Geometry: final body of the model. Coordinates: model frame, mm. Face numbers are marked on the shaded views. Round coordinates to 2 decimals unless told otherwise and drop trailing zeros. Loops run counter-clockwise (first coordinate to the right, second up) from the corner with the lowest first, then second, coordinate; pieces in that order, holes last. Notation, with made-up numbers: (44.5, 21) - (87.5, 21) arc R26 ccw to (87.5, 44) - close; hole circle Ø2 at (-28.5, -29). An arc over 180 degrees is marked (long way). Write item = value, one per line. Start each with the question number.
Item 1: Line query: line 1 (Z direction, x = -3, y = 83); line 2 (Y direction, x = -0.5, z = -2); line 3 (X direction, y = 74.5, z = -2.5). Output: solid intervals per line, ascending. Write a range as from..to.
Item 2: Draft query along Z for the marked faces 1 and 2. Return one class per face: pulls with the +Z half, pulls with the -Z half, needs draft (parallel to the pull), parting line crosses it, or undercut.
Item 3: Section A-A (y = 55). Return loops of the section in (x, z), plus the area to 3 significant figures.
Item 4: First-contact query: pin 1 (1.6 mm diameter, centred on x = -0.5, y = 5, fed in from +Z); pin 2 (4 mm diameter, centred on y = 47, z = -0.5, fed in from -X); pin 3 (1.2 mm diameter, centred on x = 0, y = 5, fed in from -Z); pin 4 (1.6 mm diameter, centred on x = -0.5, y = 4.5, fed in from -Z). Flat tips, straight axial feed; report the tip coordinate or a pass-through.
from build123d import *

# Parameters (mm, degrees)
SKETCH2_R           = 1
CUT_EXTRUDE1_DEPTH  = 5
CUT_EXTRUDE2_DEPTH  = 2.5
CUT_EXTRUDE3_DEPTH  = 5
SKETCH5_R           = 1
BOSS_EXTRUDE1_DEPTH = 4.5


with BuildPart() as part:
    # Sketch1 → Revolve1 (revolve)
    with BuildSketch(Plane.XY, mode=Mode.PRIVATE) as revolve1_sk:
        with BuildLine():
            Line((0, 0), (0, 88.2))
            ThreePointArc((0, 88.2), (-2.741592985, 87.073746186), (-3.899734916, 84.345470721))
            Line((-3.899734916, 84.345470721), (-4.65, 20))
            Line((-4.65, 20), (-4.65, 0))
            Line((-4.65, 0), (0, 0))
        make_face()
    revolve(revolve1_sk.sketch.rotate(Axis((0, 0, 0), (0, 1, 0)), 270), axis=Axis((0, 0, 0), (0, 1, 0)))

    # Sketch2 → Cut-Extrude1 (cut, symmetric)
    with BuildSketch(Plane.XY):
        with Locations((0, 5)):
            Circle(SKETCH2_R)
    extrude(amount=CUT_EXTRUDE1_DEPTH, both=True, mode=Mode.SUBTRACT)

    # Sketch3 → Cut-Extrude2 (cut, symmetric)
    with BuildSketch(Plane.XY):
        with BuildLine():
            Line((3, 0), (3, 5))
            ThreePointArc((3, 5), (2.121320344, 7.121320344), (0, 8))
            Line((0, 8), (-4.65, 8))
            Line((-4.65, 8), (-4.65, 0))
            Line((-4.65, 0), (3, 0))
        make_face()
    extrude(amount=CUT_EXTRUDE2_DEPTH, both=True, mode=Mode.SUBTRACT)

    # Sketch4 → Cut-Extrude3 (cut, symmetric)
    with BuildSketch(Plane.XY):
        with BuildLine():
            Line((-5, 5), (-8, 5))
            Line((-8, 5), (-8, -3))
            Line((-8, -3), (0, -3))
            Line((0, -3), (0, 0))
            ThreePointArc((0, 0), (-3.535533906, 1.464466094), (-5, 5))
        make_face()
    extrude(amount=CUT_EXTRUDE3_DEPTH, both=True, mode=Mode.SUBTRACT)

    # Sketch5 → Boss-Extrude1 (add, symmetric)
    with BuildSketch(Plane.XY):
        with Locations((0, 5)):
            Circle(SKETCH5_R)
    extrude(amount=BOSS_EXTRUDE1_DEPTH, both=True)


solid = part.part
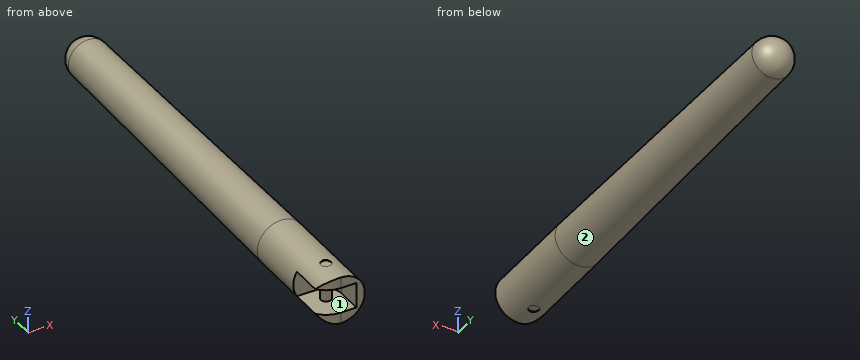
Taken from the geometry:
q1.line_1 = -2.52..2.52
q1.line_2 = 4.13..5.87, 8..87.61
q1.line_3 = -3.14..3.14
q2.face_1 = undercut
q2.face_2 = parting line crosses it
q3.outline = circle Ø8.48 at (0, 0)
q3.area = 56.5 mm^2
q4.pin_1 = 4.61
q4.pin_2 = -4.36
q4.pin_3 = -4.5
q4.pin_4 = -4.65
